from build123d import *

# Parameters (mm, degrees)
F0_W     = 24
F0_H     = 24
F0_R     = 1.35
F1_DEPTH = 4.6
F2_W     = 7.2
F2_H     = 15.2
F3_DEPTH = 4.601
F2_W_2   = 10.3
F2_H_2   = 18.5
F4_DEPTH = 2.2
F5_R     = 4


with BuildPart() as f1:
    # F0 (on Top) → F1 (new body)
    with BuildSketch(Plane.XY):
        Rectangle(F0_W, F0_H)
        with Locations((-8, -8)):
            Circle(F0_R, mode=Mode.SUBTRACT)
        with Locations((8, -8)):
            Circle(F0_R, mode=Mode.SUBTRACT)
        with Locations((-8, 8)):
            Circle(F0_R, mode=Mode.SUBTRACT)
        with Locations((8, 8)):
            Circle(F0_R, mode=Mode.SUBTRACT)
    extrude(amount=F1_DEPTH)

    # F2 (on face) → F3 (cut, through all)
    with BuildSketch(Plane.XY.offset(4.6)):
        Rectangle(F2_W, F2_H)
    extrude(amount=-F3_DEPTH, mode=Mode.SUBTRACT)

    # F2 (on face) → F4 (cut)
    with BuildSketch(Plane.XY.offset(4.6)):
        Rectangle(F2_W_2, F2_H_2)
        Rectangle(F2_W, F2_H, mode=Mode.SUBTRACT)
    extrude(amount=-F4_DEPTH, mode=Mode.SUBTRACT)

    # F5
    f5_edges = [f1.edges().sort_by_distance(p)[0] for p in [
        (-12, 12, 2.3),
        (12, 12, 2.3),
        (12, -12, 2.3),
        (-12, -12, 2.3),
    ]]
    fillet(f5_edges, radius=F5_R)


solid = f1.part
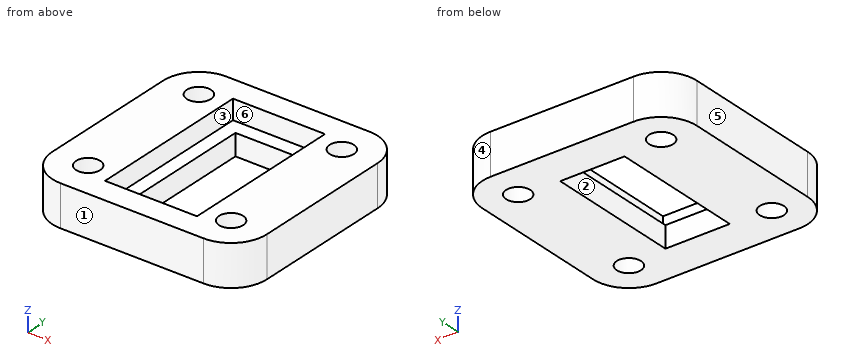
The listing builds one solid part. Answer for the finished solid, in the listing's coordinates (mm). Face numbers are marked on the shaded views. A direction names the side the tool comes from. Coordinates: 2 decimals unless noted, no trailing zeros. Order: outer loops, then holes, each group sorted by start corner. A loop starts at its lowest first (then second) coordinate and runs counter-clockwise, first axis right, second up.
Q1. A cutting plane is placed at D-D, the plane z = 0.5. Write down the section's boundary in (x, y).
Q2. A cutting plane is placed at C-C, the plane x = -1.75. Write down the section's boundary in (y, z), and give its area (3 significant figures).
Q3. Given P1, Ø12, axis at x = 5, y = -7, coming from the -Z side, flat-ended and moving along its own axis, determine where the tip first touches the part or whether it passes through.
Q4. Which of the six approach directions +Z, -Z, +X, -X, +Y, -Y give full straight-line access (tool end or side, diameter ignored) to the marked faces 1, 2 and 3?
Q5. A cutting plane is placed at A-A, the plane y = 2.5. Write down the section's boundary in (x, z).
Q6. For a pull along Y with two mould halves and no side action, classify the marked faces 4, 5 and 6 as pulls with the +Y half, pulls with the -Y half, needs draft (parallel to the pull), parting line crosses it, or undercut.
Q7. A cutting plane is placed at B-B, the plane z = 3.5. Write down the section's boundary in (x, y), and give its area (3 significant figures).
Q8. Consider line 1 (Y direction, x = 8, z = 1.25); line 2 (X direction, y = 2, z = 3.5); line 3 (Y direction, x = 1.5, z = 0.5). Determine where each line is inside the solid, lowest interval first.
Answers follow:
1. outline: (-12, -8) arc R4 ccw to (-8, -12) - (8, -12) arc R4 ccw to (12, -8) - (12, 8) arc R4 ccw to (8, 12) - (-8, 12) arc R4 ccw to (-12, 8) - close; hole circle Ø2.7 at (-8, -8); hole circle Ø2.7 at (-8, 8); hole (-3.6, -7.6) - (3.6, -7.6) - (3.6, 7.6) - (-3.6, 7.6) - close; hole circle Ø2.7 at (8, -8); hole circle Ø2.7 at (8, 8)
2. outline: (-12, 0) - (-7.6, 0) - (-7.6, 2.4) - (-9.25, 2.4) - (-9.25, 4.6) - (-12, 4.6) - close; (7.6, 0) - (12, 0) - (12, 4.6) - (9.25, 4.6) - (9.25, 2.4) - (7.6, 2.4) - close
2. area: 33.2 mm2
3. P1: stops at z = 0
4. face 1: +Z, -Z, +X, -X, -Y
4. face 2: +Z, -Z
4. face 3: +Z
5. outline: (-12, 0) - (-3.6, 0) - (-3.6, 2.4) - (-5.15, 2.4) - (-5.15, 4.6) - (-12, 4.6) - close; (3.6, 0) - (12, 0) - (12, 4.6) - (5.15, 4.6) - (5.15, 2.4) - (3.6, 2.4) - close
6. face 4: pulls with the +Y half
6. face 5: needs draft
6. face 6: undercut
7. outline: (-12, -8) arc R4 ccw to (-8, -12) - (8, -12) arc R4 ccw to (12, -8) - (12, 8) arc R4 ccw to (8, 12) - (-8, 12) arc R4 ccw to (-12, 8) - close; hole circle Ø2.7 at (-8, -8); hole circle Ø2.7 at (-8, 8); hole (-5.15, -9.25) - (5.15, -9.25) - (5.15, 9.25) - (-5.15, 9.25) - close; hole circle Ø2.7 at (8, -8); hole circle Ø2.7 at (8, 8)
7. area: 349 mm2
8. line 1: y = -12 to -9.35, -6.65 to 6.65, 9.35 to 12
8. line 2: x = -12 to -5.15, 5.15 to 12
8. line 3: y = -12 to -7.6, 7.6 to 12
